The figure shows three views and two pictorial views of one solid part (mm, origin at its lowest corner). Answer the questions. A direction names the side the tool comes from. Give positions to 0.01 mm unless a question says otherwise; leave off trailing zeros. Write each loop counter-clockwise with the first axis right and the second up, starting at its lowest first coordinate (ties: lowest second). Pieces come first, ordered by that corner, then holes. Notation, with made-up numbers: (14.25, 36) -> (43.25, 36) arc R10 ccw to (43.25, 52) -> close; hole circle Ø3 at (61.25, 2). An arc over 180 degrees is marked (long way). Answer as CSV lines item,"result". Start each with the question number.
1. The part is cut by section A-A, the plane z = 34. Determine the outline of the cut face in (x, y).
2. A tool of negligible diameter and unlimited length cuts with its end or side. For the marked faces 4, 5 and 6, from which of +Z, -Z, +X, -X, +Y, -Y can it reach the whole face along a straight path? Write none if from no direction.
3. The part is cut by section B-B, the plane x = 31. Determine the outline of the cut face in (y, z), and give its area (3 significant figures).
4. Given pin 1 (20 mm diameter, centred on x = 23.5, z = 33, fed in from -Y); pin 2 (3 mm diameter, centred on x = 15, y = 7, fed in from +Z); pin 3 (8 mm diameter, centred on x = 44.5, y = 32, fed in from +Z), each flat-ended and moving along its own axis, determine where each tip first touches the part or whether it passes through.
5. For a pull along X with two mould halves and no side action, classify the marked faces 1, 2 and 3 as pulls with the +X half, pulls with the -X half, needs draft (parallel to the pull), parting line crosses it, or undercut.
6. The part is cut by section C-C, the plane z = 19. Determine the outline of the cut face in (x, y).
7. Find the intervals of material crossed by line 1 (X direction, y = 33.5, z = 24); line 2 (Z direction, x = 24.5, y = 4.5); line 3 (Y direction, x = 27.5, z = 33), in increasing order.
8. The part is cut by section D-D, the plane y = 32. Determine the outline of the cut face in (x, z), and give its area (3 significant figures).
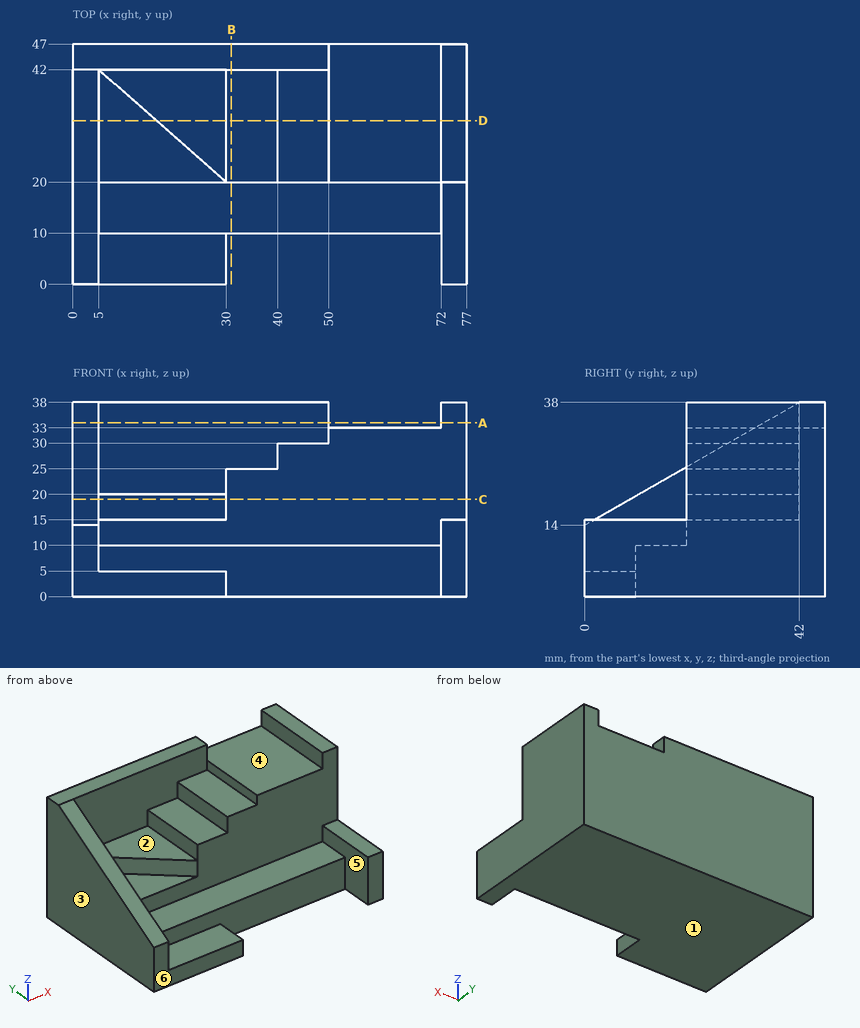
Results found:
1,outline,"(0, 35) -> (5, 35) -> (5, 42) -> (50, 42) -> (50, 47) -> (0, 47) -> close; (72, 20) -> (77, 20) -> (77, 47) -> (72, 47) -> close"
2,face 4,"+Z, +Y, -Y"
2,face 5,"+Z, -Y"
2,face 6,"+Z, -Z, +X, -X, -Y"
3,outline,"(10, 0) -> (47, 0) -> (47, 38) -> (42, 38) -> (42, 25) -> (20, 25) -> (20, 10) -> (10, 10) -> close"
3,area,"840 mm²"
4,pin 1,"stops at y = 42"
4,pin 2,"stops at z = 5"
4,pin 3,"stops at z = 30"
5,face 1,"needs draft"
5,face 2,"undercut"
5,face 3,"pulls with the -X half"
6,outline,"(0, 8.75) -> (5, 8.75) -> (5, 42) -> (30, 20) -> (77, 20) -> (77, 47) -> (0, 47) -> close"
7,line 1,"x = 0 to 5, 30 to 77"
7,line 2,"z = 0 to 5"
7,line 3,"y = 42 to 47"
8,outline,"(0, 0) -> (77, 0) -> (77, 38) -> (72, 38) -> (72, 33) -> (50, 33) -> (50, 30) -> (40, 30) -> (40, 25) -> (30, 25) -> (30, 20) -> (16.36, 20) -> (16.36, 15) -> (5, 15) -> (5, 32.29) -> (0, 32.29) -> close"
8,area,"2,070 mm²"
